The model under review builds one solid part; all positions refer to its coordinate system, in mm. Face numbers are marked on the shaded views. A direction names the side the tool comes from. Round coordinates to 2 decimals unless told otherwise and drop trailing zeros. Order: outer loops, then holes, each group sorted by start corner. A loop starts at its lowest first (then second) coordinate and runs counter-clockwise, first axis right, second up.
1) Machinability: for the marked faces 4, 5, 6 and 7, which of the approach directions +Z, -Z, +X, -X, +Y, -Y give a long, thin tool a straight path to every point of the face, cutting with its end or side? Answer none if there is none.
2) Consider section B-B (y = 8.75). Give the boundary of the cut face in (x, z) (3 decimals), then the cut area to 3 significant figures.
3) Mouldability with a two-part tool opening along X and no side actions: class the marked faces 1, 2 and 3 as pulls with the +X half, pulls with the -X half, needs draft (parallel to the pull), parting line crosses it, or undercut.
4) To check wall thickness, follow L1, parallel to Y at x = -4, z = 1.75; L2, parallel to Y at x = 2.5, z = 0.5; L3, parallel to X at y = 3.75, z = 1. State the ranges of each line that lie inside material, in increasing order.
5) Clearance check with flat-ended pins moving along their axes: P1, Ø3, axis at x = -3, z = -1, coming from the +Y side; P2, Ø1.1, axis at x = 0.5, z = 0.5, coming from the +Y side; P3, Ø1.8, axis at x = 1.5, y = 5.5, coming from the +Z side; P4, Ø5, axis at x = -4, y = 8.5, coming from the -Z side. State where each tip first meets the part, or that it passes through.
6) Consider section D-D (y = 2.25). Give the boundary of the cut face in (x, z).
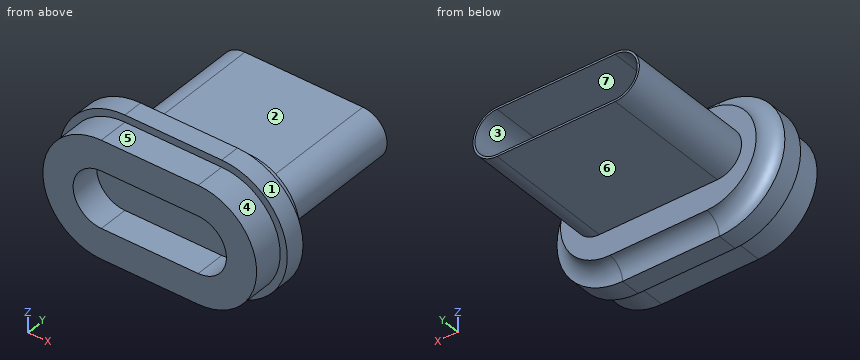
from build123d import *

# Parameters (mm, degrees)
BOSS_EXTRUDE1_DEPTH = 1.5
BOSS_EXTRUDE2_DEPTH = 1
BOSS_EXTRUDE4_DEPTH = 0.8
BOSS_EXTRUDE3_DEPTH = 6.5
FILLET1_R           = 0.8


with BuildPart() as part:
    # Sketch1 → Boss-Extrude1 (new body)
    with BuildSketch(Plane(origin=(0, 0, 0), x_dir=(1, 0, 0), z_dir=(0, 1, 0))):
        with BuildLine():
            Line((-2.4, 2.9), (2.4, 2.9))
            ThreePointArc((2.4, 2.9), (5.3, 0), (2.4, -2.9))
            Line((2.4, -2.9), (-2.4, -2.9))
            ThreePointArc((-2.4, -2.9), (-5.3, 0), (-2.4, 2.9))
        make_face()
        with BuildLine():
            Line((-2.4, 1.4), (2.4, 1.4))
            ThreePointArc((2.4, 1.4), (3.8, 0), (2.4, -1.4))
            Line((2.4, -1.4), (-2.4, -1.4))
            ThreePointArc((-2.4, -1.4), (-3.8, 0), (-2.4, 1.4))
        make_face(mode=Mode.SUBTRACT)
    extrude(amount=BOSS_EXTRUDE1_DEPTH)

    # Sketch2 → Boss-Extrude2 (add)
    with BuildSketch(Plane(origin=(0, 1.5, 0), x_dir=(1, 0, 0), z_dir=(0, 1, 0))):
        with BuildLine():
            Line((-2.4, -3.25), (2.4, -3.25))
            ThreePointArc((2.4, -3.25), (5.65, 0), (2.4, 3.25))
            Line((2.4, 3.25), (-2.4, 3.25))
            ThreePointArc((-2.4, 3.25), (-5.65, 0), (-2.4, -3.25))
        make_face()
    extrude(amount=BOSS_EXTRUDE2_DEPTH)

    # Sketch4 → Boss-Extrude4 (add)
    with BuildSketch(Plane(origin=(0, 2.5, 0), x_dir=(1, 0, 0), z_dir=(0, 1, 0))):
        with BuildLine():
            Line((-2.4, -2.45), (2.4, -2.45))
            ThreePointArc((2.4, -2.45), (4.85, 0), (2.4, 2.45))
            Line((2.4, 2.45), (-2.4, 2.45))
            ThreePointArc((-2.4, 2.45), (-4.85, 0), (-2.4, -2.45))
        make_face()
    extrude(amount=BOSS_EXTRUDE4_DEPTH)

    # Sketch3 → Boss-Extrude3 (add)
    with BuildSketch(Plane(origin=(0, 3.3, 0), x_dir=(1, 0, 0), z_dir=(0, 1, 0))):
        with BuildLine():
            Line((-2.925, 1.2), (2.925, 1.2))
            ThreePointArc((2.925, 1.2), (4.125, 0), (2.925, -1.2))
            Line((2.925, -1.2), (-2.925, -1.2))
            ThreePointArc((-2.925, -1.2), (-4.125, 0), (-2.925, 1.2))
        make_face()
        with BuildLine():
            Line((-2.925, 1.1), (2.925, 1.1))
            ThreePointArc((2.925, 1.1), (4.025, 0), (2.925, -1.1))
            Line((2.925, -1.1), (-2.925, -1.1))
            ThreePointArc((-2.925, -1.1), (-4.025, 0), (-2.925, 1.1))
        make_face(mode=Mode.SUBTRACT)
    extrude(amount=BOSS_EXTRUDE3_DEPTH)

    # Fillet1
    fillet1_edges = [part.edges().sort_by_distance(p)[0] for p in [
        (-4.85, 2.5, 0),
        (0, 2.5, -2.45),
        (4.85, 2.5, 0),
        (0, 2.5, 2.45),
    ]]
    fillet(fillet1_edges, radius=FILLET1_R - 0.0001)  # a hair under: the kernel refuses the full size


solid = part.part
Answer below:
1. face 4: +X, -Y
1. face 5: +Z, +X, -X, -Y
1. face 6: -Z, +X, -X, +Y
1. face 7: +Y
2. outline: (-2.925, -1.2) - (2.925, -1.2) arc R1.2 ccw to (2.925, 1.2) - (-2.925, 1.2) arc R1.2 ccw to start; hole (-2.925, -1.1) - (2.925, -1.1) arc R1.1 ccw to (2.925, 1.1) - (-2.925, 1.1) arc R1.1 ccw to start
2. area: 1.89 mm2
3. face 1: pulls with the +X half
3. face 2: needs draft
3. face 3: undercut
4. L1: y = 0 to 3.3
4. L2: y = 1.5 to 3.3
4. L3: x = -3.59 to -3.38, 3.38 to 3.59
5. P1: stops at y = 9.8
5. P2: stops at y = 3.3
5. P3: stops at z = 1.2
5. P4: stops at z = -1.2
6. outline: (-2.4, -3.25) - (2.4, -3.25) arc R3.25 ccw to (2.4, 3.25) - (-2.4, 3.25) arc R3.25 ccw to start
